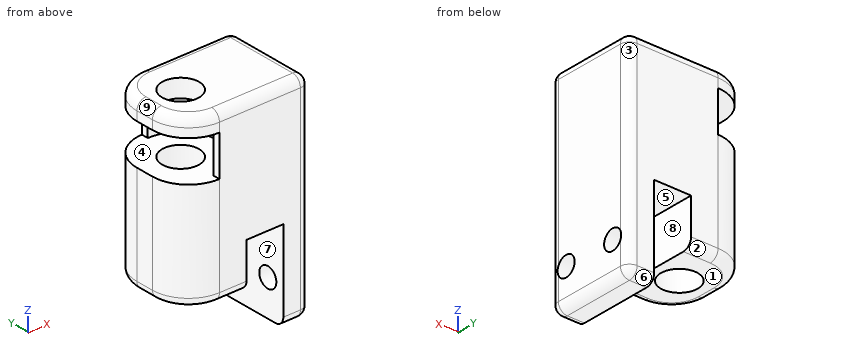
from build123d import *

# Parameters (mm, degrees)
F0_R          = 4.1
F1_DEPTH      = 34
F3_DEPTH      = 9
F4_R          = 4.1
F5_DEPTH      = 4
F6_W          = 8.2
F6_H          = 20
F7_DEPTH      = 20
F8_W          = 15.1884564608
F8_H          = 21.6641027853
F9_DEPTH      = 10
F10_R         = 2.2
F11_DEPTH     = 25
F12_T1_DEPTH  = 8.8
F12_T3_DEPTH  = 18
F12_T5_DEPTH  = 16
F12_T7_DEPTH  = 43
F12_T9_DEPTH  = 4
F12_T11_DEPTH = 11
F12_S15_W     = 2
F12_S15_H     = 2
F12_T16_DEPTH = 2
F12_S21_W     = 2
F12_S21_H     = 2
F12_T22_DEPTH = 2
F12_S27_W     = 2
F12_S27_H     = 2
F12_T28_DEPTH = 2
F12_S33_W     = 2
F12_S33_H     = 2
F12_T34_DEPTH = 2
F12_T38_ANGLE = 90
F12_T40_ANGLE = 90
F12_T42_ANGLE = 90
F12_T44_ANGLE = 90


# Not quite as in the source:
# - a fillet or chamfer that OpenCascade refuses, or shapes differently, is made with other operations: its cross-section is extruded or revolved along the edge and cut away or added


with BuildPart() as f1:
    # F0 (on Top) → F1 (new body)
    with BuildSketch(Plane.XY):
        with BuildLine():
            ThreePointArc((-8, -2), (-5.6568542495, -7.6568542495), (0, -10))
            Line((0, -10), (20, -10))
            Line((20, -10), (20, 10))
            Line((20, 10), (0, 10))
            ThreePointArc((0, 10), (-5.6568542495, 7.6568542495), (-8, 2))
            Line((-8, 2), (-8, -2))
        make_face()
        Circle(F0_R, mode=Mode.SUBTRACT)
    extrude(amount=F1_DEPTH)

    # F2 (on face) → F3 (join)
    with BuildSketch(Plane.XY.offset(34)):
        with BuildLine():
            Line((0, 10), (0, 8.5))
            ThreePointArc((0, 8.5), (8.5, 0), (0, -8.5))
            Line((0, -8.5), (0, -10))
            Line((0, -10), (20, -10))
            Line((20, -10), (20, 10))
            Line((20, 10), (0, 10))
        make_face()
    extrude(amount=F3_DEPTH)

    # F4 (on face) → F5 (join)
    with BuildSketch(Plane.XY.offset(43)):
        with BuildLine():
            Line((20, -10), (20, 10))
            Line((20, 10), (0, 10))
            ThreePointArc((0, 10), (-5.6568542495, 7.6568542495), (-8, 2))
            Line((-8, 2), (-8, -2))
            ThreePointArc((-8, -2), (-5.6568542495, -7.6568542495), (0, -10))
            Line((0, -10), (20, -10))
        make_face()
        Circle(F4_R, mode=Mode.SUBTRACT)
    extrude(amount=F5_DEPTH)

    # F6 (on face) → F7 (cut)
    with BuildSketch(Plane(origin=(0, 0, 0), x_dir=(1, 0, 0), z_dir=(0, 0, -1))):
        with Locations((10.1, 0)):
            Rectangle(F6_W, F6_H)
    extrude(amount=-F7_DEPTH, mode=Mode.SUBTRACT)

    # F8 (on face) → F9 (cut)
    with BuildSketch(Plane(origin=(0, 0, 0), x_dir=(1, 0, 0), z_dir=(0, 0, -1))):
        with Locations((-1.5942282304, 0.8320513926)):
            Rectangle(F8_W, F8_H)
    extrude(amount=-F9_DEPTH, mode=Mode.SUBTRACT)

    # F10 (on face) → F11 (cut)
    with BuildSketch(Plane(origin=(14.2, 0, 0), x_dir=(0, -1, 0), z_dir=(-1, 0, 0))):
        with Locations((6, 8)):
            Circle(F10_R)
        with Locations((-6, 8)):
            Circle(F10_R)
    extrude(amount=-F11_DEPTH, mode=Mode.SUBTRACT)

    # F12: fillet of radius 2 on 16 edges, made by hand

    # F12_s2 → F12_t1 (cut)
    with BuildSketch(Plane.YZ.offset(9.2)):
        with BuildLine():
            ThreePointArc((10, 2), (9.4142135624, 0.5857864376), (8, 0))
            Line((8, 0), (10, 0))
            Line((10, 0), (10, 2))
        make_face()
        with BuildLine():
            ThreePointArc((-10, 2), (-9.4142135624, 0.5857864376), (-8, 0))
            Line((-8, 0), (-10, 0))
            Line((-10, 0), (-10, 2))
        make_face()
    extrude(amount=F12_T1_DEPTH, mode=Mode.SUBTRACT)

    # F12_s4 → F12_t3 (cut)
    with BuildSketch(Plane.YZ):
        with BuildLine():
            ThreePointArc((10, 45), (9.4142135624, 46.4142135624), (8, 47))
            Line((8, 47), (10, 47))
            Line((10, 47), (10, 45))
        make_face()
        with BuildLine():
            ThreePointArc((-10, 45), (-9.4142135624, 46.4142135624), (-8, 47))
            Line((-8, 47), (-10, 47))
            Line((-10, 47), (-10, 45))
        make_face()
    extrude(amount=F12_T3_DEPTH, mode=Mode.SUBTRACT)

    # F12_s6 → F12_t5 (cut)
    with BuildSketch(Plane.XZ.offset(-8)):
        with BuildLine():
            ThreePointArc((20, 45), (19.4142135624, 46.4142135624), (18, 47))
            Line((18, 47), (20, 47))
            Line((20, 47), (20, 45))
        make_face()
        with BuildLine():
            ThreePointArc((20, 2), (19.4142135624, 0.5857864376), (18, 0))
            Line((18, 0), (20, 0))
            Line((20, 0), (20, 2))
        make_face()
    extrude(amount=F12_T5_DEPTH, mode=Mode.SUBTRACT)

    # F12_s8 → F12_t7 (cut)
    with BuildSketch(Plane.XY.offset(2)):
        with BuildLine():
            ThreePointArc((18, 10), (19.4142135624, 9.4142135624), (20, 8))
            Line((20, 8), (20, 10))
            Line((20, 10), (18, 10))
        make_face()
        with BuildLine():
            ThreePointArc((18, -10), (19.4142135624, -9.4142135624), (20, -8))
            Line((20, -8), (20, -10))
            Line((20, -10), (18, -10))
        make_face()
    extrude(amount=F12_T7_DEPTH, mode=Mode.SUBTRACT)

    # F12_s10 → F12_t9 (cut)
    with BuildSketch(Plane.XZ.offset(-2)):
        with BuildLine():
            ThreePointArc((-6, 10), (-7.4142135624, 10.5857864376), (-8, 12))
            Line((-8, 12), (-8, 10))
            Line((-8, 10), (-6, 10))
        make_face()
        with BuildLine():
            ThreePointArc((-6, 47), (-7.4142135624, 46.4142135624), (-8, 45))
            Line((-8, 45), (-8, 47))
            Line((-8, 47), (-6, 47))
        make_face()
    extrude(amount=F12_T9_DEPTH, mode=Mode.SUBTRACT)

    # F12_s12 → F12_t11 (cut)
    with BuildSketch(Plane.YZ):
        with BuildLine():
            ThreePointArc((-8, 10), (-9.4142135624, 10.5857864376), (-10, 12))
            Line((-10, 12), (-10, 10))
            Line((-10, 10), (-8, 10))
        make_face()
        with BuildLine():
            ThreePointArc((8, 10), (9.4142135624, 10.5857864376), (10, 12))
            Line((10, 12), (10, 10))
            Line((10, 10), (8, 10))
        make_face()
    extrude(amount=F12_T11_DEPTH, mode=Mode.SUBTRACT)


with BuildPart() as f12_tool14:
    # F12_s15 → F12_t16 (new body)
    with BuildSketch(Plane.YZ.offset(18)):
        with Locations((9, 1)):
            Rectangle(F12_S15_W, F12_S15_H)
    extrude(amount=F12_T16_DEPTH)

    # F12_s17 → F12_t18 (revolve, cut)
    with BuildSketch(Plane(origin=(18, 8, 2), x_dir=(0, -0.7071067812, 0.7071067812), z_dir=(0, 0.7071067812, 0.7071067812))):
        with BuildLine():
            ThreePointArc((0, -2), (2, 0), (0, 2))
            Line((0, 2), (0, -2))
        make_face()
    revolve(axis=Axis((18, 8, 2), (1, 0, 0)), mode=Mode.SUBTRACT)


with BuildPart() as f1_1:
    add(f1.part)

    # F12_t13: cut F12_tool14
    add(f12_tool14.part, mode=Mode.SUBTRACT)


with BuildPart() as f12_tool20:
    # F12_s21 → F12_t22 (new body)
    with BuildSketch(Plane.XY.offset(45)):
        with Locations((19, 9)):
            Rectangle(F12_S21_W, F12_S21_H)
    extrude(amount=F12_T22_DEPTH)

    # F12_s23 → F12_t24 (revolve, cut)
    with BuildSketch(Plane(origin=(18, 8, 45), x_dir=(-0.7071067812, -0.7071067812, 0), z_dir=(-0.7071067812, 0.7071067812, 0))):
        with BuildLine():
            ThreePointArc((0, -2), (2, 0), (0, 2))
            Line((0, 2), (0, -2))
        make_face()
    revolve(axis=Axis((18, 8, 45), (0, 0, 1)), mode=Mode.SUBTRACT)


with BuildPart() as f1_2:
    add(f1_1.part)

    # F12_t19: cut F12_tool20
    add(f12_tool20.part, mode=Mode.SUBTRACT)


with BuildPart() as f12_tool26:
    # F12_s27 → F12_t28 (new body)
    with BuildSketch(Plane.XY.offset(45)):
        with Locations((19, -9)):
            Rectangle(F12_S27_W, F12_S27_H)
    extrude(amount=F12_T28_DEPTH)

    # F12_s29 → F12_t30 (revolve, cut)
    with BuildSketch(Plane(origin=(18, -8, 45), x_dir=(-0.7071067812, 0.7071067812, 0), z_dir=(0.7071067812, 0.7071067812, 0))):
        with BuildLine():
            ThreePointArc((0, -2), (2, 0), (0, 2))
            Line((0, 2), (0, -2))
        make_face()
    revolve(axis=Axis((18, -8, 45), (0, 0, 1)), mode=Mode.SUBTRACT)


with BuildPart() as f1_3:
    add(f1_2.part)

    # F12_t25: cut F12_tool26
    add(f12_tool26.part, mode=Mode.SUBTRACT)


with BuildPart() as f12_tool32:
    # F12_s33 → F12_t34 (new body)
    with BuildSketch(Plane.YZ.offset(18)):
        with Locations((-9, 1)):
            Rectangle(F12_S33_W, F12_S33_H)
    extrude(amount=F12_T34_DEPTH)

    # F12_s35 → F12_t36 (revolve, cut)
    with BuildSketch(Plane(origin=(18, -8, 2), x_dir=(0, 0.7071067812, 0.7071067812), z_dir=(0, 0.7071067812, -0.7071067812))):
        with BuildLine():
            ThreePointArc((0, -2), (2, 0), (0, 2))
            Line((0, 2), (0, -2))
        make_face()
    revolve(axis=Axis((18, -8, 2), (1, 0, 0)), mode=Mode.SUBTRACT)


with BuildPart() as f1_4:
    add(f1_3.part)

    # F12_t31: cut F12_tool32
    add(f12_tool32.part, mode=Mode.SUBTRACT)

    # F12_s37 → F12_t38 (revolve, cut)
    with BuildSketch(Plane.YZ):
        with BuildLine():
            ThreePointArc((-8, 10), (-9.4142135624, 10.5857864376), (-10, 12))
            Line((-10, 12), (-10, 10))
            Line((-10, 10), (-8, 10))
        make_face()
    revolve(axis=Axis((0, -2, 10), (0, 0, -1)), revolution_arc=F12_T38_ANGLE, mode=Mode.SUBTRACT)

    # F12_s39 → F12_t40 (revolve, cut)
    with BuildSketch(Plane.XZ.offset(-2)):
        with BuildLine():
            ThreePointArc((-8, 12), (-7.4142135624, 10.5857864376), (-6, 10))
            Line((-6, 10), (-8, 10))
            Line((-8, 10), (-8, 12))
        make_face()
    revolve(axis=Axis((0, 2, 10), (0, 0, -1)), revolution_arc=F12_T40_ANGLE, mode=Mode.SUBTRACT)

    # F12_s41 → F12_t42 (revolve, cut)
    with BuildSketch(Plane.YZ):
        with BuildLine():
            ThreePointArc((10, 45), (9.4142135624, 46.4142135624), (8, 47))
            Line((8, 47), (10, 47))
            Line((10, 47), (10, 45))
        make_face()
    revolve(axis=Axis((0, 2, 47), (0, 0, 1)), revolution_arc=F12_T42_ANGLE, mode=Mode.SUBTRACT)

    # F12_s43 → F12_t44 (revolve, cut)
    with BuildSketch(Plane.XZ.offset(2)):
        with BuildLine():
            ThreePointArc((-6, 47), (-7.4142135624, 46.4142135624), (-8, 45))
            Line((-8, 45), (-8, 47))
            Line((-8, 47), (-6, 47))
        make_face()
    revolve(axis=Axis((0, -2, 47), (0, 0, 1)), revolution_arc=F12_T44_ANGLE, mode=Mode.SUBTRACT)


solid = f1_4.part
Verification items for the finished model (mm, model axes). Face numbers are marked on the shaded views. A direction names the side the tool comes from. Round coordinates to 2 decimals unless told otherwise and drop trailing zeros. Write each loop counter-clockwise with the first axis right and the second up, starting at its lowest first coordinate (ties: lowest second). Pieces come first, ordered by that corner, then holes.
(1) Section check A-A (z = 12.5). Enter the section's corners in (x, y), plus the area to 3 significant figures.
Returned:
outline: (-8, -2) arc R8 ccw to (0, -10) - (6, -10) - (6, 10) - (0, 10) arc R8 ccw to (-8, 2) - close; (14.2, -10) - (18, -10) arc R2 ccw to (20, -8) - (20, 8) arc R2 ccw to (18, 10) - (14.2, 10) - close; hole circle Ø8.2 at (0, 0)
area: 314 mm2
(2) Section check C-C (x = 2.25). Enter the section's corners in (y, z), plus the area to 3 significant figures.
Returned:
outline: (-10, 12) arc R2 ccw to (-8, 10) - (-3.43, 10) - (-3.43, 34) - (-8.2, 34) - (-8.2, 43) - (-3.43, 43) - (-3.43, 47) - (-8, 47) arc R2 ccw to (-10, 45) - close; (3.43, 10) - (8, 10) arc R2 ccw to (10, 12) - (10, 45) arc R2 ccw to (8, 47) - (3.43, 47) - (3.43, 43) - (8.2, 43) - (8.2, 34) - (3.43, 34) - close
area: 397 mm2
(3) Mould release check, pull along X, two halves, no side actions. Record for the marked faces 6, 7, 8 and 9: pulls with the +X half, pulls with the -X half, needs draft (parallel to the pull), parting line crosses it, or undercut.
Returned:
face 6: needs draft
face 7: undercut
face 8: undercut
face 9: pulls with the -X half
(4) Material ranges on line 1 (Y direction, x = 16.45, z = 8); line 2 (X direction, y = 0, z = 28.5); line 3 (Z direction, x = 16.7, y = 6), recorded low to high.
Returned:
line 1: y = -10 to -8.2, -3.8 to 3.8, 8.2 to 10
line 2: x = -8 to -4.1, 4.1 to 20
line 3: z = 0 to 5.8, 10.2 to 47
(5) Depth check by flat-ended pin: pin 1 Ø4 at (x, y) = (4.5, -0.5) entering from -Z; pin 2 Ø7.5 at (x, y) = (0, 0) entering from +Z; pin 3 Ø1.6 at (y, z) = (9, 40.5) entering from -X; pin 4 Ø2 at (y, z) = (6, 12) entering from -X. Enter the tip coordinate at first touch or a pass-through.
Returned:
pin 1: stops at z = 10
pin 2: passes through
pin 3: stops at x = 0
pin 4: stops at x = -7.42
(6) Section check D-D (z = 3). Enter the section's corners in (x, y).
Returned:
outline: (14.2, -10) - (18, -10) arc R2 ccw to (20, -8) - (20, 8) arc R2 ccw to (18, 10) - (14.2, 10) - close
(7) Section check B-B (y = 0). Enter the section's corners in (x, z), plus the area to 3 significant figures.
Returned:
outline: (-8, 12) arc R2 ccw to (-6, 10) - (-4.1, 10) - (-4.1, 34) - (-8, 34) - close; (-8, 43) - (-4.1, 43) - (-4.1, 47) - (-6, 47) arc R2 ccw to (-8, 45) - close; (4.1, 10) - (6, 10) - (6, 20) - (14.2, 20) - (14.2, 0) - (18, 0) arc R2 ccw to (20, 2) - (20, 45) arc R2 ccw to (18, 47) - (4.1, 47) - (4.1, 43) - (8.5, 43) - (8.5, 34) - (4.1, 34) - close
area: 630 mm2
(8) Access from +Z, -Z, +X, -X, +Y, -Y to the whole of each face (thin tool, end or side, straight path). Record for the marked faces 1, 2, 3, 4 and 5.
Returned:
face 1: -Z, -X, +Y, -Y
face 2: -Z, -X, +Y
face 3: +Z, -Z, +X, +Y
face 4: -X
face 5: -Z, +Y, -Y
